Autodesk Inventor part; units mm, degrees
ref_plane "YZ Plane" through (0, 0, 0) normal (1, 0, 0) x (0, 1, 0)
ref_plane "XZ Plane" through (0, 0, 0) normal (0, 1, 0) x (-1, 0, 0)
ref_plane "XY Plane" through (0, 0, 0) normal (0, 0, 1) x (1, 0, 0)
sketch "Sketch1" plane through (0, 0, 0) normal (0, 1, 0) x (-1, 0, 0)
  circle A0 centre (0, 0) radius 7.5
  circle A1 centre (0, 0) radius 5
  circle A2 centre (0, 0) radius 4
  circle A3 centre (0, 0) radius 3
  circle A4 centre (0, 0) radius 6
  dimension "d0" = 15
  dimension "d1" = 10
  dimension "d2" = 8
  dimension "d7" = 6
  dimension "d8" = 12
extrude "Extrusion1" add sketch "Sketch1" along normal blind 8 contours A0
extrude "Extrusion2" add sketch "Sketch1" against normal blind 44 contours A1 | A2
extrude "Extrusion3" add sketch "Sketch1" along normal blind 4 contours A0 | A1 | A2 | A4
sketch "Sketch2" plane through (0, -44, 0) normal (0, -1, 0) x (1, 0, 0)
  circle A0 centre (0, 0) radius 5
  line L0 (5, 0) -> (2.5, -4.3301)
  line L1 (2.5, -4.3301) -> (-2.5, -4.3301)
  line L2 (-2.5, -4.3301) -> (-5, 0)
  line L3 (-5, 0) -> (-2.5, 4.3301)
  line L4 (-2.5, 4.3301) -> (2.5, 4.3301)
  line L5 (2.5, 4.3301) -> (5, 0)
  circle A1 centre (0, 0) radius 5
  dimension "d11" = 10
extrude "Extrusion4" cut sketch "Sketch2" against normal blind 5 contours L5 A0 | A0 L0 | L4 A0 | A0 L1 | L3 A0 | A0 L2
properties part number "vacuum-gear-shaft"
Read the model definition and answer for the solid it produces. Units are mm, in the model's axes. A direction names the side the tool comes from. Give positions to 0.01 mm unless a question says otherwise; leave off trailing zeros. Order: outer loops, then holes, each group sorted by start corner. A loop starts at its lowest first (then second) coordinate and runs counter-clockwise, first axis right, second up.
(1) Find section B-B (y = -31.5). Give the vertices of the cut face in (x, z).
(2) Straight lines are drawn through the part: L1, parallel to X at y = -4, z = -0.25; L2, parallel to Z at x = 0, y = 7.1; L3, parallel to Z at x = 0, y = -16.5. For each, find the intervals that lie inside material, in ascending order.
(3) Given pin 1 (3.5 mm diameter, centred on x = -1.5, z = -1.5, fed in from +Y); pin 2 (5.5 mm diameter, centred on x = 0, y = -42.5, fed in from -Z); pin 3 (1.2 mm diameter, centred on x = -4, z = -3, fed in from -Y), each flat-ended and moving along its own axis, determine where each tip first touches the part or whether it passes through.
(4) Find section D-D (x = -4.25). Give the vertices of the cut face in (y, z).
(5) For faces 5 (the flat face through (3, 4, -1)), 6 (the flat face through (-3.77, -41.54, 2.13)), 7 (the flat face through (0, -42, 4.33)), 8 (the flat face through (3.77, -41.54, -2.13)), 9 (the flat face through (3.73, -41.54, 2.2)), determine the directions among +Z, -Z, +X, -X, +Y, -Y from which every point of the face is accessible in a straight line to the end or side of a thin tool.
(6) Find section A-A (x = 0). Give the vertices of the cut face in (y, z), plus the area to 3 significant figures.
(7) Find section C-C (z = 3.5). Give the vertices of the cut face in (x, y).
(8) For a pull along Z with two mould halves and no side action, classify faces 1 (the cylindrical face through (1.08, -19.23, -4.88)), 2 (the flat face through (-2, 0, -5)), 3 (the cylindrical face through (6, 6, 0)), 4 (the flat face through (-3.73, -41.54, -2.2)) as released by +Z, released by -Z, zero draft, split by the parting line, or undercut.
Result sheet:
1. outline: circle Ø10 at (0, 0); hole circle Ø6 at (0, 0)
2. L1: x = -4.99 to -2.99, 2.99 to 4.99
2. L2: z = -7.5 to -6, 6 to 7.5
2. L3: z = -5 to -3, 3 to 5
3. pin 1: stops at y = 4
3. pin 2: stops at z = -4.33
3. pin 3: stops at y = -39
4. outline: (-44, -1.3) - (-39, -1.3) - (-39, -2.63) - (0, -2.63) - (0, -6.18) - (8, -6.18) - (8, -4.24) - (4, -4.24) - (4, 4.24) - (8, 4.24) - (8, 6.18) - (0, 6.18) - (0, 2.63) - (-39, 2.63) - (-39, 1.3) - (-44, 1.3) - close
5. face 5: +Y
5. face 6: +Z, -X, -Y
5. face 7: +Z, +X, -X, -Y
5. face 8: -Z, +X, -Y
5. face 9: +Z, +X, -Y
6. outline: (-44, -4.33) - (-39, -4.33) - (-39, -5) - (0, -5) - (0, -7.5) - (8, -7.5) - (8, -6) - (4, -6) - (4, -3) - (-44, -3) - close; (-44, 3) - (4, 3) - (4, 6) - (8, 6) - (8, 7.5) - (0, 7.5) - (0, 5) - (-39, 5) - (-39, 4.33) - (-44, 4.33) - close
6. area: 217 mm2
7. outline: (-6.63, 0) - (-3.57, 0) - (-3.57, -39) - (-2.98, -39) - (-2.98, -44) - (2.98, -44) - (2.98, -39) - (3.57, -39) - (3.57, 0) - (6.63, 0) - (6.63, 8) - (4.87, 8) - (4.87, 4) - (-4.87, 4) - (-4.87, 8) - (-6.63, 8) - close
8. face 1: split by the parting line
8. face 2: zero draft
8. face 3: undercut
8. face 4: released by -Z
